The model under review builds one solid part; all positions refer to its coordinate system, in mm. Coordinates: 2 decimals unless noted, no trailing zeros. Loops run counter-clockwise (first coordinate to the right, second up) from the corner with the lowest first, then second, coordinate; pieces in that order, holes last. Notation, with made-up numbers: M 10,-6 L 17,-6 A29 ccw 17,32 Z; hole C -40,69 d10. An arc over 180 degrees is marked long. One line per item, written item: value.
```python
from build123d import *

# Parameters (mm, degrees)
CROQUIS1_R                   = 50
SALIENTE_EXTRUIR1_DEPTH      = 5
TALADRO_DE_MARGEN_PARA_M51_D = 5.5
MATRIZC1_COUNT               = 6


with BuildPart() as part:
    # Croquis1 → Saliente-Extruir1 (new body)
    with BuildSketch(Plane(origin=(0, 0, 0), x_dir=(1, 0, 0), z_dir=(0, 1, 0))):
        Circle(CROQUIS1_R)
    extrude(amount=SALIENTE_EXTRUIR1_DEPTH)

    # Taladro de margen para M51 (through all)
    with Locations(Plane(origin=(0, 0, 0), x_dir=(-1, 0, 0), z_dir=(0, -1, 0))):
        with Locations((0, 44.178034415)):
            taladro_de_margen_para_m51 = Hole(TALADRO_DE_MARGEN_PARA_M51_D / 2)

    # MatrizC1: Taladro de margen para M51 ×6 about axis
    matrizc1_axis = Axis((0, 0, 0), (0, 1, 0))
    for i in range(1, MATRIZC1_COUNT):
        add(taladro_de_margen_para_m51.rotate(matrizc1_axis, i * 360 / MATRIZC1_COUNT), mode=Mode.SUBTRACT)


solid = part.part
```
(1) Insertion check: pin 1 Ø5 at (x, z) = (0, 44.18) entering from +Y; pin 2 Ø2 at (y, z) = (3, -19.5) entering from -X. Each pin has a flat end and moves straight along its axis. Give the tip position at first contact, or say it passes through.
Checks:
pin 1: through
pin 2: x = -46.45
(2) Add section B-B on y = 2.8. State the section outline as (x, z) points.
Checks:
outline: C 0,0 d100; hole C -38.26,-22.09 d5.5; hole C -38.26,22.09 d5.5; hole C 0,-44.18 d5.5; hole C 0,44.18 d5.5; hole C 38.26,-22.09 d5.5; hole C 38.26,22.09 d5.5
(3) To check wall thickness, follow L1, parallel to Z at x = 0, y = 1.25; L2, parallel to X at y = 4.75, z = 24.5; L3, parallel to X at y = 2.45, z = -28. State the ranges of each line that lie inside material, in increasing order. Write a range as [from, to].
Checks:
L1: [-50, -46.93], [-41.43, 41.43], [46.93, 50]
L2: [-43.59, -39.58], [-36.94, 36.94], [39.58, 43.59]
L3: [-41.42, 41.42]
(4) Add section A-A on x = 0. State the section outline as (y, z) points.
Checks:
outline: M 0,-50 L 5,-50 L 5,-46.93 L 0,-46.93 Z; M 0,-41.43 L 5,-41.43 L 5,41.43 L 0,41.43 Z; M 0,46.93 L 5,46.93 L 5,50 L 0,50 Z
(5) Draft analysis for pull direction Z (two halves, no side actions). For faces 1 (the face through (47.69, 2.46, -15.02)), 2 (the face through (-35.51, 2.53, -21.97)), 3 (the face through (-1, 0, -1)), state which applies: pulls with the +Z half, pulls with the -Z half, needs draft (parallel to the pull), parting line crosses it, or undercut.
Checks:
face 1: parting line crosses it
face 2: undercut
face 3: needs draft
